Autodesk Inventor part; units mm, degrees
ref_plane "YZ Plane" through (0, 0, 0) normal (1, 0, 0) x (0, 1, 0)
ref_plane "XZ Plane" through (0, 0, 0) normal (0, 1, 0) x (-1, 0, 0)
ref_plane "XY Plane" through (0, 0, 0) normal (0, 0, 1) x (1, 0, 0)
sketch "スケッチ1" plane through (0, 0, 0) normal (0, 0, 1) x (1, 0, 0)
  line L0 (-5, 19) -> (5, 19)
  line L1 (5, 19) -> (5, -19)
  line L2 (5, -19) -> (-5, -19)
  line L3 (-5, -19) -> (-5, 19)
  line L4 (-5, 19) -> (5, -19) construction
  line L5 (5, 19) -> (-5, -19) construction
  point P0 (0, 0)
  dimension "d0" = 10
  dimension "d1" = 38
extrude "押し出し1" add sketch "スケッチ1" along normal blind 1.5
sketch "スケッチ2" plane through (0, 0, 1.5) normal (0, 0, 1) x (1, 0, 0)
  line L0 (5, 19) -> (-5, 19)
  line L1 (5, -19) -> (5, 19)
  line L2 (-5, -19) -> (5, -19)
  point P0 (0, 0)
  point P1 (0, -14)
  point P2 (0, 2)
  dimension "d6" = 5
  dimension "d7" = 5
  dimension "d8" = 16
hole "穴1" at (0, -14, 1.5) at (0, 2, 1.5) direction (0, 0, -1) diameter 2.1 end through all
sketch "スケッチ3" plane through (0, 0, 1.5) normal (0, 0, 1) x (1, 0, 0)
  line L0 (5, 19) -> (-5, 19)
  line L1 (5, -19) -> (5, 19)
  point P0 (0, 0)
  point P1 (0, 14)
  dimension "d16" = 5
  dimension "d17" = 5
hole "穴2" at (0, 14, 1.5) direction (0, 0, -1) diameter 3.1 end through all
properties part number "servo catch front c"
The listing builds one solid part. Answer for the finished solid, in the listing's coordinates (mm). Coordinates: 2 decimals unless noted, no trailing zeros. Order: outer loops, then holes, each group sorted by start corner. A loop starts at its lowest first (then second) coordinate and runs counter-clockwise, first axis right, second up. Notation, with made-up numbers: M 22,39 L 36,39 A9 ccw 36,45 Z; hole C 6.25,26.5 d6. An arc over 180 degrees is marked long. Answer as a JSON object with one key per item and string values. Group by question number.
1. A flat-ended cylindrical pin translates along its axis: P1, Ø2.5, axis at x = 0, y = 14, coming from the +Z side. Find the tip coordinate at first contact, or state that the pin passes through.
2. Section A-A on y = 14 is taken. Write down the section's boundary in (x, z).
3. Section C-C on y = -14 is taken. Write down the section's boundary in (x, z), then the cut area to 4 significant figures.
4. Determine the mould class of faces 1 (the flat face through (5, 0, 1)), 2 (the cylindrical face through (-0.05, -12.95, 0.74)), 3 (the flat face through (0, 19, 1)), 4 (the flat face through (-5, 0, 1)) for opening direction X: released by +X, released by -X, zero draft, split by the parting line, or undercut.
5. Section B-B on z = 0.75 is taken. Write down the section's boundary in (x, y), then the cut area to 3 significant figures.
6. Straight lines are drawn through the part: line 1 (Y direction, x = 0, z = 0.3); line 2 (X direction, y = 14, z = 0.9); line 3 (Y direction, x = -0.75, z = 0.9). For each, find the intervals that lie inside material, in ascending order.
Values follow:
{
 "1": {"P1": "through"},
 "2": {"outline": "M -5,0 L -1.55,0 L -1.55,1.5 L -5,1.5 Z; M 1.55,0 L 5,0 L 5,1.5 L 1.55,1.5 Z"},
 "3": {"outline": "M -5,0 L -1.05,0 L -1.05,1.5 L -5,1.5 Z; M 1.05,0 L 5,0 L 5,1.5 L 1.05,1.5 Z", "area": "11.85 mm2"},
 "4": {"face 1": "released by +X", "face 2": "undercut", "face 3": "zero draft", "face 4": "released by -X"},
 "5": {"outline": "M -5,-19 L 5,-19 L 5,19 L -5,19 Z; hole C 0,14 d3.1; hole C 0,-14 d2.1; hole C 0,2 d2.1", "area": "366 mm2"},
 "6": {"line 1": "-19 to -15.05, -12.95 to 0.95, 3.05 to 12.45, 15.55 to 19", "line 2": "-5 to -1.55, 1.55 to 5", "line 3": "-19 to -14.73, -13.27 to 1.27, 2.73 to 12.64, 15.36 to 19"}
}
